CAD build for the part. Positions are in the model's coordinates, mm. A direction names the side the tool comes from. Round coordinates to 2 decimals unless told otherwise and drop trailing zeros. Loops run counter-clockwise (first coordinate to the right, second up) from the corner with the lowest first, then second, coordinate; pieces in that order, holes last. Notation, with made-up numbers: M -5.5,62.25 L 17.5,62.25 A20 ccw 17.5,75.25 Z; hole C -4.5,-24 d10. An arc over 180 degrees is marked long. One line per item, written item: value. Start each with the question number.
Autodesk Inventor part; units mm, degrees
ref_plane "YZ Plane" through (0, 0, 0) normal (1, 0, 0) x (0, 1, 0)
ref_plane "XZ Plane" through (0, 0, 0) normal (0, 1, 0) x (-1, 0, 0)
ref_plane "XY Plane" through (0, 0, 0) normal (0, 0, 1) x (1, 0, 0)
sketch "Sketch1" plane through (0, 0, 0) normal (0, 1, 0) x (-1, 0, 0)
  circle A0 centre (0, 0) radius 5.5563
  dimension "d0" = 11.1125
extrude "Extrusion1" add sketch "Sketch1" along normal blind 76.2
sketch "Sketch2" plane through (0, 0, 0) normal (0, -1, 0) x (1, 0, 0)
  circle A0 centre (0, 0) radius 2
  dimension "d3" = 4
sketch "Sketch3" plane through (0, 76.2, 0) normal (0, 1, 0) x (1, 0, 0)
  circle A0 centre (0, 0) radius 2
  dimension "d4" = 4
extrude "Extrusion2" cut sketch "Sketch3" against normal blind 7
extrude "Extrusion3" cut sketch "Sketch2" against normal blind 7
equation "\"d3\" = m3_heat_set_insert"
equation "\"d4\" = m3_heat_set_insert"
equation "\"d5\" = m3_heat_set_depth"
equation "\"d7\" = m3_heat_set_depth"
equation "\"m3_heat_set_insert\" = 4"
equation "\"m3_clearance\" = 3.4"
equation "\"m3_heat_set_depth\" = 7"
equation "\"hardboard_thickness\" = 5"
equation "\"robot_diameter\" = 354"
equation "\"motor_centerline_height\" = 13"
properties part number "3inch_standoff"
(1) Probe L1, parallel to Z at x = 0, y = 72.75; L2, parallel to Y at x = 1.25, z = 0.75; L3, parallel to X at y = 8, z = -0.25. List the from-to ranges inside material, lowest first.
(2) Which spindle directions (+Z, -Z, +X, -X, +Y, -Y) get a long thin tool onto all of the face, cutting with end or side? Do faces 5 (the flat face through (0.1, 0, -2.4)), 6 (the cylindrical face through (0, 73, 2)). Say none if no direction does.
(3) Flat gauge pins, fed straight in: P1, Ø1.5, axis at y = 11, z = -3, coming from the -X side; P2, Ø2.5, axis at x = 0, z = 0, coming from the +Y side; P3, Ø3, axis at x = 0, z = 0, coming from the -Y side. Where does each tip first touch, or does it go through?
(4) Slice it at D-D, the plane x = 3.75. List the corners of the cut face in (y, z), and give its area (3 significant figures).
(5) Slice it at B-B, the plane x = 0. List the corners of the cut face in (y, z), and give its area (3 significant figures).
(6) Slice it at A-A, the plane z = 0. List the corners of the cut face in (x, y).
(7) Mould opens along Z. For faces 1 (the cylindrical face through (0, 3, -2)), 2 (the cylindrical face through (1.204, 37.567, 5.424)), 3 (the flat face through (0.1, 76.2, -2.4)), 4 (the flat face through (0, 7, 0)) say: pulls with the +Z half, pulls with the -Z half, needs draft (parallel to the pull), parting line crosses it, or undercut.
(8) Slice it at C-C, the plane y = 19. List the corners of the cut face in (x, z).
Check result:
1. L1: z = -5.56 to -2, 2 to 5.56
1. L2: y = 7 to 69.2
1. L3: x = -5.55 to 5.55
2. face 5: +Z, -Z, +X, -X, -Y
2. face 6: +Y
3. P1: stops at x = -5.08
3. P2: stops at y = 69.2
3. P3: stops at y = 7
4. outline: M 0,-4.1 L 76.2,-4.1 L 76.2,4.1 L 0,4.1 Z
4. area: 625 mm^2
5. outline: M 0,-5.56 L 76.2,-5.56 L 76.2,-2 L 69.2,-2 L 69.2,2 L 76.2,2 L 76.2,5.56 L 0,5.56 L 0,2 L 7,2 L 7,-2 L 0,-2 Z
5. area: 791 mm^2
6. outline: M -5.56,0 L -2,0 L -2,7 L 2,7 L 2,0 L 5.56,0 L 5.56,76.2 L 2,76.2 L 2,69.2 L -2,69.2 L -2,76.2 L -5.56,76.2 Z
7. face 1: undercut
7. face 2: parting line crosses it
7. face 3: needs draft
7. face 4: undercut
8. outline: C 0,0 d11.11
